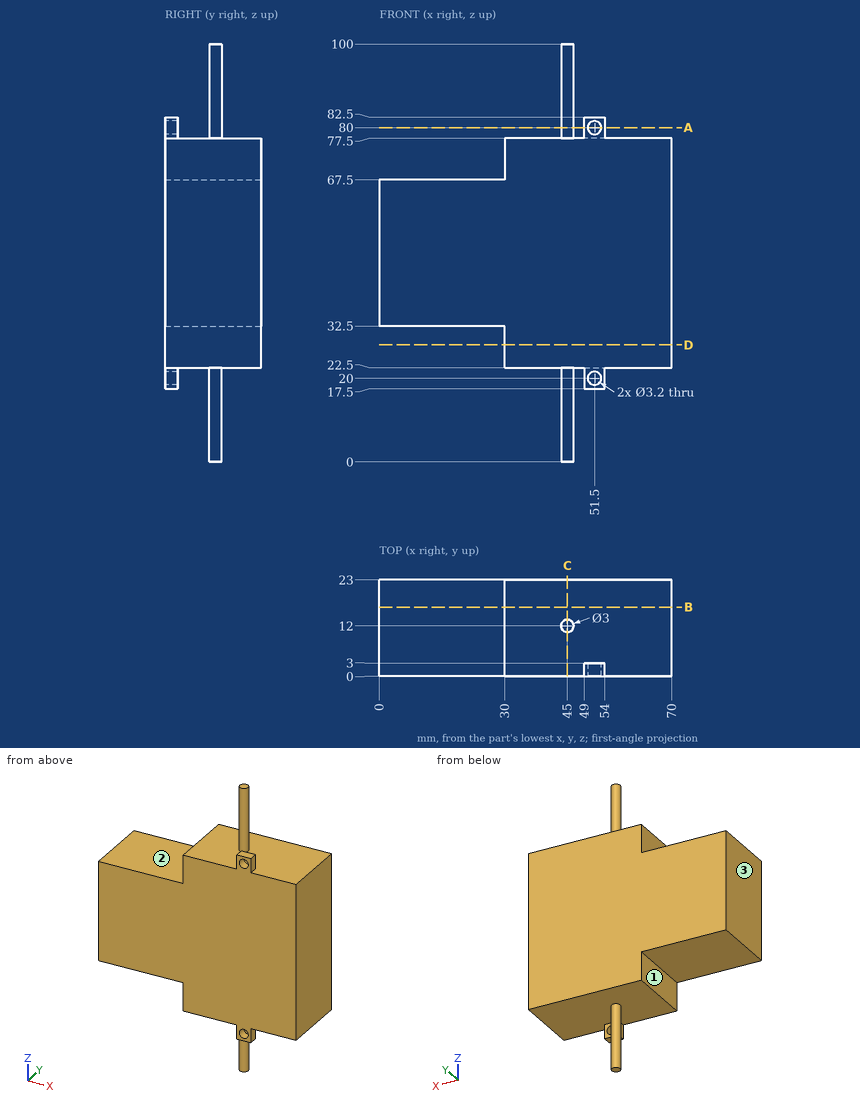
Answer from the drawing. Dimensions are ordinates in mm from the lowest x, y and z of the part. A direction names the side the tool comes from. Round coordinates to 2 decimals unless told otherwise and drop trailing zeros. Write each loop counter-clockwise with the first axis right and the second up, starting at its lowest first coordinate (ties: lowest second). Pieces come first, ordered by that corner, then holes.
1. The part is cut by section B-B, the plane y = 16.5. Determine the outline of the cut face in (x, z).
2. The part is cut by section C-C, the plane x = 45. Determine the outline of the cut face in (y, z), then the cut area to 3 significant figures.
3. The part is cut by section D-D, the plane z = 28. Determine the outline of the cut face in (x, y), then the cut area to 3 significant figures.
4. Which of the six approach directions +Z, -Z, +X, -X, +Y, -Y give full straight-line access (tool end or side, diameter ignored) to the marked faces 1, 2 and 3?
5. The part is cut by section A-A, the plane z = 80. Determine the outline of the cut face in (x, y), then the cut area to 3 significant figures.
6. Straight lines are drawn through the part: L1, parallel to Z at x = 51.5, y = 1.25; L2, parallel to X at y = 1.5, z = 80; L3, parallel to Z at x = 52.5, y = 2.25. For each, find the intervals that lie inside material, in ascending order.
7. Given pin 1 Ø7 at (x, y) = (8, 8) entering from +Z; pin 2 Ø1.5 at (x, y) = (32, 10.5) entering from +Z; pin 3 Ø12 at (x, y) = (52.5, 8) entering from -Z, each flat-ended and moving along its own axis, determine where each tip first touches the part or whether it passes through.
Values:
1. outline: (0, 32.5) - (30, 32.5) - (30, 22.5) - (70, 22.5) - (70, 77.5) - (30, 77.5) - (30, 67.5) - (0, 67.5) - close
2. outline: (0, 22.5) - (10.5, 22.5) - (10.5, 0) - (13.5, 0) - (13.5, 22.5) - (23, 22.5) - (23, 77.5) - (13.5, 77.5) - (13.5, 100) - (10.5, 100) - (10.5, 77.5) - (0, 77.5) - close
2. area: 1,400 mm2
3. outline: (30, 0) - (70, 0) - (70, 23) - (30, 23) - close
3. area: 920 mm2
4. face 1: -Z, -X, +Y, -Y
4. face 2: +Z, -X, +Y, -Y
4. face 3: +Z, -Z, -X, +Y, -Y
5. outline: circle Ø3 at (45, 12); (49, 0) - (49.9, 0) - (49.9, 3) - (49, 3) - close; (53.1, 0) - (54, 0) - (54, 3) - (53.1, 3) - close
5. area: 12.5 mm2
6. L1: z = 17.5 to 18.4, 21.6 to 78.4, 81.6 to 82.5
6. L2: x = 49 to 49.9, 53.1 to 54
6. L3: z = 17.5 to 18.75, 21.25 to 78.75, 81.25 to 82.5
7. pin 1: stops at z = 67.5
7. pin 2: stops at z = 77.5
7. pin 3: stops at z = 17.5
